Design review of the part built by this model. Coordinates are the model's own, in mm. A direction names the side the tool comes from. Give positions to 0.01 mm unless a question says otherwise; leave off trailing zeros. Write each loop counter-clockwise with the first axis right and the second up, starting at its lowest first coordinate (ties: lowest second). Pieces come first, ordered by that corner, then holes. Notation, with made-up numbers: (56, 7) -> (77, 7) arc R11 ccw to (77, 16) -> close; hole circle Ø11 at (9.5, -24). An arc over 180 degrees is marked (long way). Write each question's results on one line, items separated by ' | '. Start each with the question number.
(1) To check wall thickness, follow probe 1 along Z at (x, y) = (1.5, 2.75); probe 2 along Z at (x, y) = (-1, -1); probe 3 along Y at (x, z) = (0, 3.45) (3 decimals). State the ranges of each line that lie inside material, in increasing order.
(2) Mouldability with a two-part tool opening along X and no side actions: class faces 1 (the face through (0, -3.1, 2)), 2 (the face through (-3.1, 0, 2)), 3 (the face through (-2.58, 1.77, 3.6)) as released by +X, released by -X, zero draft, split by the parting line, or undercut.
(3) Take a section at B-B (y = 0). State the section outline as (x, z) points (3 decimals), plus the area to 3 significant figures.
(4) Clearance check with flat-ended pins moving along their axes: pin 1 (3 mm diameter, centred on y = -1, z = 3, fed in from +X); pin 2 (0.9 mm diameter, centred on x = -3.5, z = 0.5, fed in from +Y); pin 3 (1 mm diameter, centred on x = 3.5, y = 2, fed in from +Z); pin 4 (2 mm diameter, centred on x = -2, y = -2.5, fed in from +Z). State where each tip first meets the part, or that it passes through.
(5) For faces 4 (the face through (-2, 2, 3.8)), 5 (the face through (2.43, 1.714, 3.603)), 6 (the face through (0, 3.1, 2)), 7 (the face through (0, -2, 0.2)), 8 (the face through (0, 2, 0.2)), list the 3-axis set-ups (+Z, -Z, +X, -X, +Y, -Y) from which the entire face can be reached by the end or side of a thin tool; tool diameter is ignored.
(6) Take a section at D-D (x = -2). State the section outline as (y, z) points (3 decimals), plus the area to 3 significant figures.
(7) Take a section at C-C (z = 4.1). State the section outline as (x, y) points (3 decimals), plus the area to 3 significant figures.
from build123d import *

# Parameters (mm, degrees)
ESQUISSE1_W                         = 6.2
ESQUISSE1_H                         = 6.2
BOSS_EXTRU_1_DEPTH                  = 2.95
BOSS_EXTRU_2_DEPTH                  = 0.3
ESQUISSE3_W                         = 0.2
ESQUISSE3_H                         = 2.65
ENL_V_MAT_EXTRU_1_DEPTH             = 8.494831552
ESQUISSE4_W                         = 3.79
ESQUISSE4_H                         = 1.325
ENL_V_MAT_EXTRU_2_DEPTH             = 0.2
ESQUISSE5_W                         = 3.79
ESQUISSE5_H                         = 1.325
ENL_V_MAT_EXTRU_3_DEPTH             = 0.2
ESQUISSE6_W                         = 0.3475
ESQUISSE6_H                         = 0.71
ENL_V_MAT_EXTRU_4_DEPTH             = 0.5
ESQUISSE7_W                         = 0.5
ESQUISSE7_H                         = 0.71
ENL_V_MAT_EXTRU_5_DEPTH             = 0.3475
ESQUISSE8_W                         = 0.3475
ESQUISSE8_H                         = 0.71
ENL_V_MAT_EXTRU_6_DEPTH             = 0.5
ESQUISSE9_W                         = 0.3475
ESQUISSE9_H                         = 0.71
ENL_V_MAT_EXTRU_7_DEPTH             = 0.5
BOSS_EXTRU_3_DEPTH                  = 0.15
DIAM_TRE_DU_PER_AGE_3_5_3_5_1_D     = 3.5
DIAM_TRE_DU_PER_AGE_3_5_3_5_1_DEPTH = 0.15
ESQUISSE13_W                        = 0.6
ESQUISSE13_H                        = 0.4
ESQUISSE14_W                        = 0.6
ESQUISSE14_H                        = 0.4
ESQUISSE15_W                        = 0.6
ESQUISSE15_H                        = 0.4
ESQUISSE16_W                        = 0.6
ESQUISSE16_H                        = 0.4
ESQUISSE17_W                        = 1.625
ESQUISSE17_H                        = 1.75
NERVURE1_START                      = -0.35
NERVURE1_DEPTH                      = 0.7
NERVURE2_START                      = -0.35
NERVURE2_DEPTH                      = 0.7
NERVURE3_START                      = -0.35
NERVURE3_DEPTH                      = 0.7
NERVURE4_START                      = -0.35
NERVURE4_DEPTH                      = 0.7
CONG_1_R                            = 0.095
CONG_2_R                            = 0.245
CONG_3_R                            = 0.75


# Read off the part's stored shape, not the designer's step: Nervure1, Nervure2, Nervure3, Nervure4
with BuildPart() as part:
    # Esquisse1 → Boss.-Extru.1 (new body)
    with BuildSketch(Plane(origin=(0, 0, 0.3), x_dir=(-1, 0, 0), z_dir=(0, 0, -1))):
        Rectangle(ESQUISSE1_W, ESQUISSE1_H)
    extrude(amount=-BOSS_EXTRU_1_DEPTH)

    # Esquisse2 → Boss.-Extru.2 (add)
    with BuildSketch(Plane(origin=(0, 0, 0.3), x_dir=(-1, 0, 0), z_dir=(0, 0, -1))):
        Polygon((-2.9, 1.575), (-2.605, 1.575), (-2.605, 2.9), (2.605, 2.9), (2.605, 1.575), (2.9, 1.575), (2.9, -1.575), (2.605, -1.575), (2.605, -2.9), (-2.605, -2.9), (-2.605, -1.575), (-2.9, -1.575), align=None)
    extrude(amount=BOSS_EXTRU_2_DEPTH)

    # Esquisse3 → Enlèv. mat.-Extru.1 (cut, through all)
    with BuildSketch(Plane.ZY.offset(2.9)):
        with Locations((0.1, 0)):
            Rectangle(ESQUISSE3_W, ESQUISSE3_H)
    extrude(amount=-ENL_V_MAT_EXTRU_1_DEPTH, mode=Mode.SUBTRACT)

    # Esquisse4 → Enlèv. mat.-Extru.2 (cut)
    with BuildSketch(Plane(origin=(0, 0, 0), x_dir=(-1, 0, 0), z_dir=(0, 0, -1))):
        with Locations((0, -2.2375)):
            Rectangle(ESQUISSE4_W, ESQUISSE4_H)
    extrude(amount=-ENL_V_MAT_EXTRU_2_DEPTH, mode=Mode.SUBTRACT)

    # Esquisse5 → Enlèv. mat.-Extru.3 (cut)
    with BuildSketch(Plane(origin=(0, 0, 0), x_dir=(-1, 0, 0), z_dir=(0, 0, -1))):
        with Locations((0, 2.2375)):
            Rectangle(ESQUISSE5_W, ESQUISSE5_H)
    extrude(amount=-ENL_V_MAT_EXTRU_3_DEPTH, mode=Mode.SUBTRACT)

    # Esquisse6 → Enlèv. mat.-Extru.4 (cut)
    with BuildSketch(Plane(origin=(0, 0, 0.3), x_dir=(-1, 0, 0), z_dir=(0, 0, -1))):
        with Locations((2.92625, -2.25)):
            Rectangle(ESQUISSE6_W, ESQUISSE6_H)
    extrude(amount=-ENL_V_MAT_EXTRU_4_DEPTH, mode=Mode.SUBTRACT)

    # Esquisse7 → Enlèv. mat.-Extru.5 (cut)
    with BuildSketch(Plane.ZY.offset(3.1)):
        with Locations((0.55, 2.25)):
            Rectangle(ESQUISSE7_W, ESQUISSE7_H)
    extrude(amount=-ENL_V_MAT_EXTRU_5_DEPTH, mode=Mode.SUBTRACT)

    # Esquisse8 → Enlèv. mat.-Extru.6 (cut)
    with BuildSketch(Plane(origin=(0, 0, 0.3), x_dir=(-1, 0, 0), z_dir=(0, 0, -1))):
        with Locations((-2.92625, -2.25)):
            Rectangle(ESQUISSE8_W, ESQUISSE8_H)
    extrude(amount=-ENL_V_MAT_EXTRU_6_DEPTH, mode=Mode.SUBTRACT)

    # Esquisse9 → Enlèv. mat.-Extru.7 (cut)
    with BuildSketch(Plane(origin=(0, 0, 0.3), x_dir=(-1, 0, 0), z_dir=(0, 0, -1))):
        with Locations((-2.92625, 2.25)):
            Rectangle(ESQUISSE9_W, ESQUISSE9_H)
    extrude(amount=-ENL_V_MAT_EXTRU_7_DEPTH, mode=Mode.SUBTRACT)

    # Esquisse10 → Boss.-Extru.3 (add)
    with BuildSketch(Plane.XY.offset(3.25)):
        with BuildLine():
            Line((1.446061231, -2.85), (-1.446061231, -2.85))
            ThreePointArc((-1.446061231, -2.85), (-1.540929561, -2.8838105), (-1.593030615, -2.97))
            ThreePointArc((-1.593030615, -2.97), (-1.64513167, -3.0561895), (-1.74, -3.09))
            Line((-1.74, -3.09), (-3.09, -3.09))
            Line((-3.09, -3.09), (-3.09, -1.74))
            ThreePointArc((-3.09, -1.74), (-3.0561895, -1.64513167), (-2.97, -1.593030615))
            ThreePointArc((-2.97, -1.593030615), (-2.8838105, -1.540929561), (-2.85, -1.446061231))
            Line((-2.85, -1.446061231), (-2.85, 1.446061231))
            ThreePointArc((-2.85, 1.446061231), (-2.8838105, 1.540929561), (-2.97, 1.593030615))
            ThreePointArc((-2.97, 1.593030615), (-3.0561895, 1.64513167), (-3.09, 1.74))
            Line((-3.09, 1.74), (-3.09, 3.09))
            Line((-3.09, 3.09), (-1.733938769, 3.09))
            ThreePointArc((-1.733938769, 3.09), (-1.639070439, 3.0561895), (-1.586969385, 2.97))
            ThreePointArc((-1.586969385, 2.97), (-1.53486833, 2.8838105), (-1.44, 2.85))
            Line((-1.44, 2.85), (1.44, 2.85))
            ThreePointArc((1.44, 2.85), (1.53486833, 2.8838105), (1.586969385, 2.97))
            ThreePointArc((1.586969385, 2.97), (1.639070439, 3.0561895), (1.733938769, 3.09))
            Line((1.733938769, 3.09), (3.09, 3.09))
            Line((3.09, 3.09), (3.09, 1.74))
            ThreePointArc((3.09, 1.74), (3.0561895, 1.64513167), (2.97, 1.593030615))
            ThreePointArc((2.97, 1.593030615), (2.8838105, 1.540929561), (2.85, 1.446061231))
            Line((2.85, 1.446061231), (2.85, -1.44))
            ThreePointArc((2.85, -1.44), (2.8838105, -1.53486833), (2.97, -1.586969385))
            ThreePointArc((2.97, -1.586969385), (3.0561895, -1.639070439), (3.09, -1.733938769))
            Line((3.09, -1.733938769), (3.09, -3.09))
            Line((3.09, -3.09), (1.74, -3.09))
            ThreePointArc((1.74, -3.09), (1.64513167, -3.0561895), (1.593030615, -2.97))
            ThreePointArc((1.593030615, -2.97), (1.540929561, -2.8838105), (1.446061231, -2.85))
        make_face()
    extrude(amount=BOSS_EXTRU_3_DEPTH)

    # Diamètre du perçage Ø3.5 (3.5)1
    with Locations(Plane.XY.offset(3.4)):
        with Locations((0, 0)):
            Hole(DIAM_TRE_DU_PER_AGE_3_5_3_5_1_D / 2, depth=DIAM_TRE_DU_PER_AGE_3_5_3_5_1_DEPTH)

    # Esquisse13 → Révolution1 (revolve)
    with BuildSketch(Plane.XZ.offset(2.3), mode=Mode.PRIVATE) as r_volution1_sk:
        with Locations((-2, 3.6)):
            Rectangle(ESQUISSE13_W, ESQUISSE13_H)
    revolve(r_volution1_sk.sketch.rotate(Axis((-2.3, -2.3, 3.8), (0, 0, -1)), 180), axis=Axis((-2.3, -2.3, 3.8), (0, 0, -1)))

    # Esquisse14 → Révolution2 (revolve)
    with BuildSketch(Plane.XZ.offset(-2.3), mode=Mode.PRIVATE) as r_volution2_sk:
        with Locations((2.6, 3.6)):
            Rectangle(ESQUISSE14_W, ESQUISSE14_H)
    revolve(r_volution2_sk.sketch.rotate(Axis((2.3, 2.3, 3.8), (0, 0, -1)), 180), axis=Axis((2.3, 2.3, 3.8), (0, 0, -1)))

    # Esquisse15 → Révolution3 (revolve)
    with BuildSketch(Plane.XZ.offset(2.3), mode=Mode.PRIVATE) as r_volution3_sk:
        with Locations((2.6, 3.6)):
            Rectangle(ESQUISSE15_W, ESQUISSE15_H)
    revolve(r_volution3_sk.sketch.rotate(Axis((2.3, -2.3, 3.8), (0, 0, -1)), 180), axis=Axis((2.3, -2.3, 3.8), (0, 0, -1)))

    # Esquisse16 → Révolution4 (revolve)
    with BuildSketch(Plane.XZ.offset(-2.3), mode=Mode.PRIVATE) as r_volution4_sk:
        with Locations((-2, 3.6)):
            Rectangle(ESQUISSE16_W, ESQUISSE16_H)
    revolve(r_volution4_sk.sketch.rotate(Axis((-2.3, 2.3, 3.8), (0, 0, -1)), 180), axis=Axis((-2.3, 2.3, 3.8), (0, 0, -1)))

    # Esquisse17 → Révolution5 (revolve)
    with BuildSketch(Plane.XZ):
        with Locations((0.8125, 4.125)):
            Rectangle(ESQUISSE17_W, ESQUISSE17_H)
    revolve(axis=Axis((0, 0, 5), (0, 0, -1)))

    # Nervure1 outline → Nervure1 (add)
    with BuildSketch(Plane(origin=(0, -2.25, 0), x_dir=(1, 0, 0), z_dir=(0, 1, 0)).offset(NERVURE1_START)):
        with BuildLine():
            Line((4.5, -0.15), (4.5, 0))
            Line((4.5, 0), (3.29447192, 0))
            Line((3.29447192, 0), (3.179694562, -0.65))
            Line((3.179694562, -0.65), (2.7525, -0.65))
            Line((2.7525, -0.65), (2.7525, -0.8))
            Line((2.7525, -0.8), (3.1, -0.8))
            ThreePointArc((3.1, -0.8), (3.257459887, -0.742700251), (3.34126743, -0.597603136))
            Line((3.34126743, -0.597603136), (3.420305438, -0.15))
            Line((3.420305438, -0.15), (4.5, -0.15))
        make_face()
    extrude(amount=NERVURE1_DEPTH)

    # Nervure2 outline → Nervure2 (add)
    with BuildSketch(Plane(origin=(0, 2.25, 0), x_dir=(1, 0, 0), z_dir=(0, 1, 0)).offset(NERVURE2_START)):
        with BuildLine():
            Line((4.5, -0.15), (4.5, 0))
            Line((4.5, 0), (3.29447192, 0))
            Line((3.29447192, 0), (3.179694562, -0.65))
            Line((3.179694562, -0.65), (2.7525, -0.65))
            Line((2.7525, -0.65), (2.7525, -0.8))
            Line((2.7525, -0.8), (3.1, -0.8))
            ThreePointArc((3.1, -0.8), (3.257459887, -0.742700251), (3.34126743, -0.597603136))
            Line((3.34126743, -0.597603136), (3.420305438, -0.15))
            Line((3.420305438, -0.15), (4.5, -0.15))
        make_face()
    extrude(amount=NERVURE2_DEPTH)

    # Nervure3 outline → Nervure3 (add)
    with BuildSketch(Plane(origin=(0, -2.25, 0), x_dir=(1, 0, 0), z_dir=(0, 1, 0)).offset(NERVURE3_START)):
        with BuildLine():
            Line((-3.179694562, -0.65), (-3.29447192, 0))
            Line((-3.29447192, 0), (-4.5, 0))
            Line((-4.5, 0), (-4.5, -0.15))
            Line((-4.5, -0.15), (-3.420305438, -0.15))
            Line((-3.420305438, -0.15), (-3.34126743, -0.597603136))
            ThreePointArc((-3.34126743, -0.597603136), (-3.257459887, -0.742700251), (-3.1, -0.8))
            Line((-3.1, -0.8), (-2.7525, -0.8))
            Line((-2.7525, -0.8), (-2.7525, -0.65))
            Line((-2.7525, -0.65), (-3.179694562, -0.65))
        make_face()
    extrude(amount=NERVURE3_DEPTH)

    # Nervure4 outline → Nervure4 (add)
    with BuildSketch(Plane.XZ.offset(-2.25).offset(NERVURE4_START)):
        with BuildLine():
            Line((-4.5, 0.15), (-4.5, 0))
            Line((-4.5, 0), (-3.29447192, 0))
            Line((-3.29447192, 0), (-3.179694562, 0.65))
            Line((-3.179694562, 0.65), (-2.7525, 0.65))
            Line((-2.7525, 0.65), (-2.7525, 0.8))
            Line((-2.7525, 0.8), (-3.1, 0.8))
            ThreePointArc((-3.1, 0.8), (-3.257459887, 0.742700251), (-3.34126743, 0.597603136))
            Line((-3.34126743, 0.597603136), (-3.420305438, 0.15))
            Line((-3.420305438, 0.15), (-4.5, 0.15))
        make_face()
    extrude(amount=NERVURE4_DEPTH)

    # Congé1
    cong_1_edges = [part.edges().sort_by_distance(p)[0] for p in [
        (-1.625, 0, 5),
        (-1.625, 0, 3.25),
        (3.420305438, -2.25, 0.15),
        (3.179694562, -2.25, 0.65),
        (3.420305438, 2.25, 0.15),
        (3.179694562, 2.25, 0.65),
        (-3.179694562, -2.25, 0.65),
        (-3.420305438, -2.25, 0.15),
        (-3.420305438, 2.25, 0.15),
        (-3.179694562, 2.25, 0.65),
    ]]
    fillet(cong_1_edges, radius=CONG_1_R)

    # Congé2
    cong_2_edges = [part.edges().sort_by_distance(p)[0] for p in [
        (3.29447192, -2.25, 0),
        (3.29447192, 2.25, 0),
        (-3.29447192, -2.25, 0),
        (-3.29447192, 2.25, 0),
    ]]
    fillet(cong_2_edges, radius=CONG_2_R)

    # Congé3
    cong_3_edges = [part.edges().sort_by_distance(p)[0] for p in [
        (3.09, -3.09, 3.325),
        (3.09, 3.09, 3.325),
        (-3.09, 3.09, 3.325),
        (-3.09, -3.09, 3.325),
    ]]
    fillet(cong_3_edges, radius=CONG_3_R)


solid = part.part
Report:
1) probe 1: 0.2 to 3.4 | probe 2: 0.2 to 5 | probe 3: -1.625 to 1.625
2) face 1: zero draft | face 2: released by -X | face 3: undercut
3) outline: (-3.1, 0.3) -> (-2.9, 0.3) -> (-2.9, 0.2) -> (2.9, 0.2) -> (2.9, 0.3) -> (3.1, 0.3) -> (3.1, 3.25) -> (2.85, 3.25) -> (2.85, 3.4) -> (1.75, 3.4) -> (1.75, 3.25) -> (1.72, 3.25) arc R0.095 cw to (1.625, 3.345) -> (1.625, 4.905) arc R0.095 ccw to (1.53, 5) -> (-1.53, 5) arc R0.095 ccw to (-1.625, 4.905) -> (-1.625, 3.345) arc R0.095 cw to (-1.72, 3.25) -> (-1.75, 3.25) -> (-1.75, 3.4) -> (-2.85, 3.4) -> (-2.85, 3.25) -> (-3.1, 3.25) -> close | area: 24.9 mm2
4) pin 1: x = 3.1 | pin 2: y = 3.1 | pin 3: z = 3.4 | pin 4: z = 3.8
5) face 4: +Z, +X, -X, +Y, -Y | face 5: +Z | face 6: +Z, -Z, +X, -X, +Y | face 7: -Z, -Y | face 8: -Z, +Y
6) outline: (-3.1, 0.3) -> (-2.9, 0.3) -> (-2.9, 0) -> (-1.325, 0) -> (-1.325, 0.2) -> (1.325, 0.2) -> (1.325, 0) -> (2.9, 0) -> (2.9, 0.3) -> (3.1, 0.3) -> (3.1, 3.25) -> (3.09, 3.25) -> (3.09, 3.4) -> (2.82, 3.4) -> (2.82, 3.8) -> (1.78, 3.8) -> (1.78, 3.4) -> (-1.78, 3.4) -> (-1.78, 3.8) -> (-2.82, 3.8) -> (-2.82, 3.4) -> (-3.09, 3.4) -> (-3.09, 3.25) -> (-3.1, 3.25) -> close | area: 21.3 mm2
7) outline: circle Ø3.25 at (0, 0) | area: 8.30 mm2
